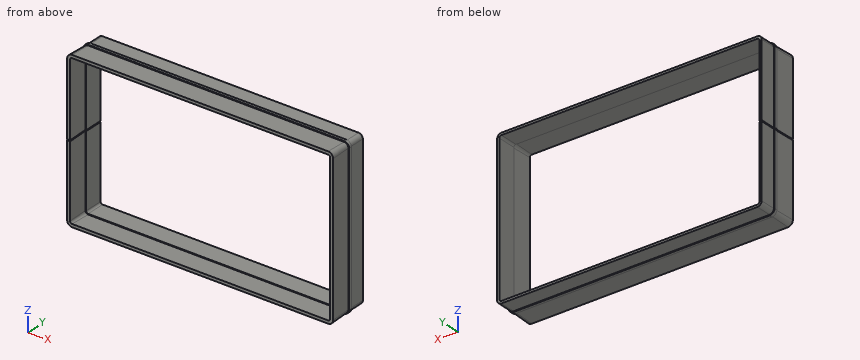
from build123d import *


with BuildPart() as part:
    # Sweep1: sweep along a path in Sketch1
    with BuildLine(Plane(origin=(0, 0, 0), x_dir=(1, 0, 0), z_dir=(0, 1, 0))) as sweep1_path:
        Line((-131, 1), (-131, 74))
        ThreePointArc((-131, 74), (-130.414213562, 75.414213562), (-129, 76))
        Line((-129, 76), (129, 76))
        ThreePointArc((129, 76), (130.414213562, 75.414213562), (131, 74))
        Line((131, 74), (131, -74))
        ThreePointArc((131, -74), (130.414213562, -75.414213562), (129, -76))
        Line((129, -76), (-129, -76))
        ThreePointArc((-129, -76), (-130.414213562, -75.414213562), (-131, -74))
        Line((-131, -74), (-131, 0))
    # Sketch2 → Sweep1 (sweep)
    with BuildSketch(Plane.XY):
        Polygon((-131, 0), (-131, -19), (-131.75, -19), (-131, -40), (-134, -40), (-133.25, -19), (-134, -19), (-134, -16), (-133.25, -16), (-133.25, 0), align=None)
    sweep(path=sweep1_path.line)


solid = part.part
Could you check a few things on this model? Use its own coordinates, in mm. Round coordinates to 2 decimals unless told otherwise and drop trailing zeros. Write each loop counter-clockwise with the first axis right and the second up, starting at its lowest first coordinate (ties: lowest second). Pieces come first, ordered by that corner, then holes. Notation, with made-up numbers: (-2.75, 23.25) - (37.25, 23.25) arc R17 ccw to (37.25, 53.25) - close; hole circle Ø11 at (-39.5, 48.5). An arc over 180 degrees is marked (long way). Use a Markdown table: item, result.
Q1. For pin 1 (15 mm diameter, centred on x = -29.5, y = -5.5, fed in from +Z); pin 2 (8 mm diameter, centred on x = 23.5, y = -32.5, fed in from +Z) (3 decimals); pin 3 (2.5 mm diameter, centred on x = -132, y = -25.5, fed in from +Z), each with a flat end and sliding along its axis, tell me the tip position at first contact or that it passes through.
Output values:
| item | result |
|---|---|
| pin 1 | z = 78.25 |
| pin 2 | z = 78.875 |
| pin 3 | z = 78.13 |
Q2. I want a section at A-A (z = 27.5). List the corners of the cut face in (x, y) for me, plus the area to 4 significant figures.
Output values:
| item | result |
|---|---|
| outline | (-134, -40) - (-131, -40) - (-131.75, -19) - (-131, -19) - (-131, 0) - (-133.25, 0) - (-133.25, -16) - (-134, -16) - (-134, -19) - (-133.25, -19) - close; (131, -40) - (134, -40) - (133.25, -19) - (134, -19) - (134, -16) - (133.25, -16) - (133.25, 0) - (131, 0) - (131, -19) - (131.75, -19) - close |
| area | 184.5 mm2 |
Q3. I want a section at D-D (y = -36). List the corners of the cut face in (x, z) for me.
Output values:
| item | result |
|---|---|
| outline | (-133.86, -74) arc R4.86 ccw to (-129, -78.86) - (129, -78.86) arc R4.86 ccw to (133.86, -74) - (133.86, 74) arc R4.86 ccw to (129, 78.86) - (-129, 78.86) arc R4.86 ccw to (-133.86, 74) - (-133.86, 0) - (-131.14, 0) - (-131.14, 74) arc R2.14 cw to (-129, 76.14) - (129, 76.14) arc R2.14 cw to (131.14, 74) - (131.14, -74) arc R2.14 cw to (129, -76.14) - (-129, -76.14) arc R2.14 cw to (-131.14, -74) - (-131.14, -1) - (-133.86, -1) - close |
Q4. I want a section at B-B (x = 92.5). List the corners of the cut face in (y, z) for me.
Output values:
| item | result |
|---|---|
| outline | (-40, -79) - (-19, -78.25) - (-19, -79) - (-16, -79) - (-16, -78.25) - (0, -78.25) - (0, -76) - (-19, -76) - (-19, -76.75) - (-40, -76) - close; (-40, 76) - (-19, 76.75) - (-19, 76) - (0, 76) - (0, 78.25) - (-16, 78.25) - (-16, 79) - (-19, 79) - (-19, 78.25) - (-40, 79) - close |
Q5. Please list where these lines run through material, in increasing order: L1, parallel to Z at x = 93.5, y = -12.5; L2, parallel to Z at x = 28, y = -17.5; L3, parallel to X at y = -2, z = 36.
Output values:
| item | result |
|---|---|
| L1 | -78.25 to -76, 76 to 78.25 |
| L2 | -79 to -76, 76 to 79 |
| L3 | -133.25 to -131, 131 to 133.25 |
Q6. I want a section at C-C (y = -10). List the corners of the cut face in (x, z) for me.
Output values:
| item | result |
|---|---|
| outline | (-133.25, -74) arc R4.25 ccw to (-129, -78.25) - (129, -78.25) arc R4.25 ccw to (133.25, -74) - (133.25, 74) arc R4.25 ccw to (129, 78.25) - (-129, 78.25) arc R4.25 ccw to (-133.25, 74) - (-133.25, 0) - (-131, 0) - (-131, 74) arc R2 cw to (-129, 76) - (129, 76) arc R2 cw to (131, 74) - (131, -74) arc R2 cw to (129, -76) - (-129, -76) arc R2 cw to (-131, -74) - (-131, -1) - (-133.25, -1) - close |
